Can you work these out from the model? Positions are in its coordinate system, mm. Round coordinates to 2 decimals unless told otherwise and drop trailing zeros. Write each loop counter-clockwise with the first axis right and the second up, starting at its lowest first coordinate (ties: lowest second). Pieces come first, ordered by that corner, then holes. Notation, with made-up numbers: M 78,-37.75 L 137,-37.75 A34 cw 137,-1.75 Z; hole C 17.5,81 d1. An arc over 180 degrees is marked long. Answer as a JSON object with one key per item and string values. Group by question number.
1) I'm going to push flat-ended pins straight in: pin 1 Ø5.5 at (x, z) = (222.5, 0) entering from +Y; pin 2 Ø5 at (y, z) = (3, 53) entering from +X; pin 3 Ø8 at (x, y) = (66.5, 4.5) entering from +Z; pin 4 Ø8 at (x, y) = (68.5, 3) entering from +Z. Where does each tip first touch, or does it pass through?
2) Suppose I cut it at A-A, the plane x = 0. Write out the boundary of the cut face in (y, z).
3) Suppose I cut it at C-C, the plane z = 88.5. Write out the boundary of the cut face in (x, y), and give its area (3 significant figures).
4) Suppose I cut it at B-B, the plane y = -2.25. Write out the boundary of the cut face in (x, z), and give its area (3 significant figures).
5) Please list where these lines run through material, in increasing order: L1, parallel to X at y = -3.75, z = 0; L2, parallel to X at y = 3.25, z = -38.5; L3, parallel to X at y = 2.5, z = -16. Write a range as [from, to].
6) Suppose I cut it at D-D, the plane z = 179. Write out the boundary of the cut face in (x, y).
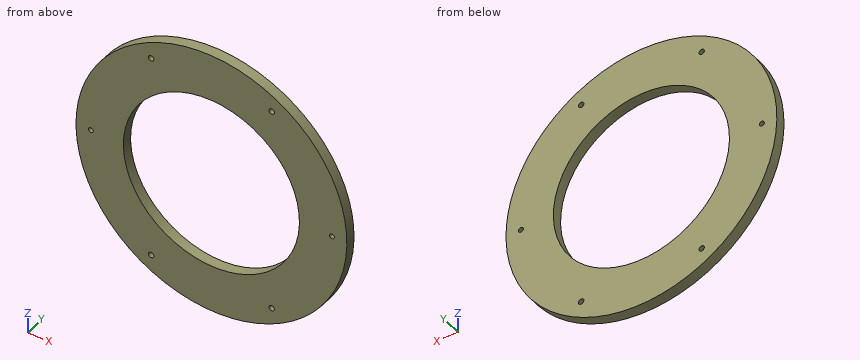
from build123d import *

# Parameters (mm, degrees)
SKETCH1_R           = 250
SKETCH1_R_2         = 162.5
BOSS_EXTRUDE1_DEPTH = 9.5
SKETCH2_R           = 5
SKETCH2_R_2         = 4.5
CUT_EXTRUDE1_DEPTH  = 355.063553617


with BuildPart() as part:
    # Sketch1 → Boss-Extrude1 (new, symmetric)
    with BuildSketch(Plane(origin=(0, 0, 0), x_dir=(1, 0, 0), z_dir=(0, 1, 0))):
        with Locations(Location((0, 0, 0), (0, 0, 270))):
            Circle(SKETCH1_R)
        with Locations(Location((0, 0, 0), (0, 0, 270))):
            Circle(SKETCH1_R_2, mode=Mode.SUBTRACT)
    extrude(amount=BOSS_EXTRUDE1_DEPTH, both=True)

    # Sketch2 → Cut-Extrude1 (cut, through all)
    with BuildSketch(Plane(origin=(0, 9.5, 0), x_dir=(1, 0, 0), z_dir=(0, 1, 0))):
        with Locations(Location((-111.25, 192.690652342, 0), (0, 0, 270))):
            Circle(SKETCH2_R)
        with Locations(Location((111.25, 192.690652342, 0), (0, 0, 270))):
            Circle(SKETCH2_R)
        with Locations(Location((222.5, 0, 0), (0, 0, 270))):
            Circle(SKETCH2_R_2)
        with Locations(Location((-111.25, -192.690652342, 0), (0, 0, 90))):
            Circle(SKETCH2_R)
        with Locations(Location((-222.5, 0, 0), (0, 0, 90))):
            Circle(SKETCH2_R_2)
        with Locations(Location((111.25, -192.690652342, 0), (0, 0, 90))):
            Circle(SKETCH2_R)
    extrude(amount=-CUT_EXTRUDE1_DEPTH, mode=Mode.SUBTRACT)


solid = part.part
Results:
{
 "1": {"pin 1": "through", "pin 2": "x = 244.85", "pin 3": "z = 242.06", "pin 4": "z = 241.54"},
 "2": {"outline": "M -9.5,-250 L 9.5,-250 L 9.5,-162.5 L -9.5,-162.5 Z; M -9.5,162.5 L 9.5,162.5 L 9.5,250 L -9.5,250 Z"},
 "3": {"outline": "M -233.81,-9.5 L -136.29,-9.5 L -136.29,9.5 L -233.81,9.5 Z; M 136.29,-9.5 L 233.81,-9.5 L 233.81,9.5 L 136.29,9.5 Z", "area": "3,710 mm^2"},
 "4": {"outline": "C 0,0 d500; hole C -222.5,0 d9; hole C 0,0 d325; hole C -111.25,-192.69 d10; hole C -111.25,192.69 d10; hole C 111.25,-192.69 d10; hole C 111.25,192.69 d10; hole C 222.5,0 d9", "area": "113,000 mm^2"},
 "5": {"L1": "[-250, -227], [-218, -162.5], [162.5, 218], [227, 250]", "L2": "[-247.02, -157.87], [157.87, 247.02]", "L3": "[-249.49, -161.71], [161.71, 249.49]"},
 "6": {"outline": "M -174.53,-9.5 L 174.53,-9.5 L 174.53,9.5 L -174.53,9.5 Z"}
}
